Geometry check sheet. Reference: the model listing, model coordinates, mm. Face numbers are marked on the shaded views. A direction names the side the tool comes from. Round coordinates to 2 decimals unless told otherwise and drop trailing zeros. Order: outer loops, then holes, each group sorted by start corner. A loop starts at its lowest first (then second) coordinate and runs counter-clockwise, first axis right, second up. Notation, with made-up numbers: M 21.5,42.5 L 49.5,42.5 A15 ccw 49.5,52.5 Z; hole C 11.5,-26 d1. An arc over 180 degrees is marked long. Return JSON: item names as keys, results as strings. Group by question number.
```python
from build123d import *

# Parameters (mm, degrees)
SKETCH1_W               = 41.91
SKETCH1_H               = 82.55
BOSS_EXTRUDE1_DEPTH     = 58.674
SKETCH2_R               = 20.32
BOSS_EXTRUDE2_DEPTH     = 76.2
SKETCH3_R               = 18.415
BOSS_EXTRUDE3_DEPTH     = 101.6
SKETCH4_R               = 9.9949
BOSS_EXTRUDE4_DEPTH     = 19.05
CUT_EXTRUDE1_DEPTH      = 19.05
CUT_EXTRUDE1_DEPTH_BACK = 19.05
SKETCH6_R               = 3.175
SKETCH7_W               = 18
SKETCH7_H               = 18
BOSS_EXTRUDE5_DEPTH     = 20
CUT_EXTRUDE2_DEPTH      = 20
CUT_EXTRUDE2_DEPTH_BACK = 20
SKETCH8_R               = 3.175


with BuildPart() as part:
    # Sketch1 → Boss-Extrude1 (new body)
    with BuildSketch(Plane.XY):
        with Locations((0, 41.275)):
            Rectangle(SKETCH1_W, SKETCH1_H)
    extrude(amount=BOSS_EXTRUDE1_DEPTH)

    # Sketch2 → Boss-Extrude2 (add)
    with BuildSketch(Plane.XY.offset(58.674)):
        with Locations(Location((0, 62.23, 0), (0, 0, 90))):
            Circle(SKETCH2_R)
    extrude(amount=BOSS_EXTRUDE2_DEPTH)

    # Sketch3 → Boss-Extrude3 (add)
    with BuildSketch(Plane.XY.offset(58.674)):
        with Locations(Location((0, 19.05, 0), (0, 0, 180))):
            Circle(SKETCH3_R)
    extrude(amount=BOSS_EXTRUDE3_DEPTH)

    # Sketch4 → Boss-Extrude4 (add)
    with BuildSketch(Plane.XY.offset(160.274)):
        with Locations(Location((0, 22.225, 0), (0, 0, 180))):
            Circle(SKETCH4_R)
    extrude(amount=BOSS_EXTRUDE4_DEPTH)

    # Sketch6 → Cut-Extrude1 (cut, two sides: drawn at the far end of the back side and taken through both)
    with BuildSketch(Plane(origin=(0, 0, 0), x_dir=(0, 0, -1), z_dir=(1, 0, 0)).offset(-CUT_EXTRUDE1_DEPTH_BACK)):
        with Locations(Location((-170.324, 22.225, 0), (0, 0, 180))):
            Circle(SKETCH6_R)
    extrude(amount=CUT_EXTRUDE1_DEPTH + CUT_EXTRUDE1_DEPTH_BACK, mode=Mode.SUBTRACT)

    # Sketch7 → Boss-Extrude5 (add)
    with BuildSketch(Plane(origin=(0, 0, 0), x_dir=(-1, 0, 0), z_dir=(0, 0, -1))):
        with Locations((0, 24)):
            Rectangle(SKETCH7_W, SKETCH7_H)
    extrude(amount=BOSS_EXTRUDE5_DEPTH)

    # Sketch8 → Cut-Extrude2 (cut, two sides: drawn at the far end of the back side and taken through both)
    with BuildSketch(Plane.ZY.offset(9).offset(-CUT_EXTRUDE2_DEPTH_BACK)):
        with Locations(Location((-12, 24, 0), (0, 0, 180))):
            Circle(SKETCH8_R)
    extrude(amount=CUT_EXTRUDE2_DEPTH + CUT_EXTRUDE2_DEPTH_BACK, mode=Mode.SUBTRACT)


solid = part.part
```
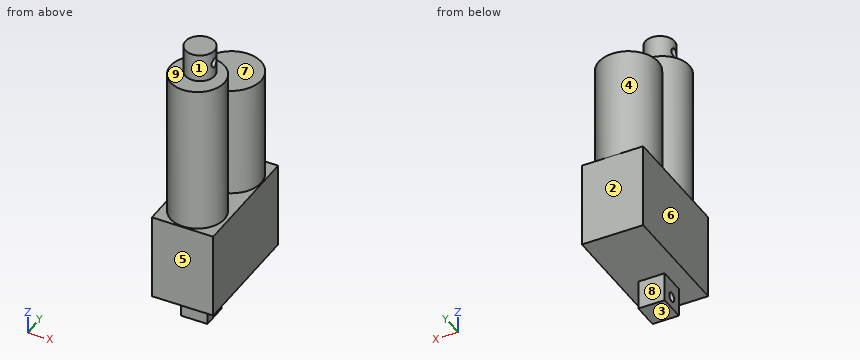
Q1. Section check A-A on z = -12. Record the cut outline in (x, y) (3 decimals), plus the area to 3 significant figures.
Q2. Section check C-C on y = 62.23. Record the cut outline in (x, z) (3 decimals), plus the area to 3 significant figures.
Q3. Depth check by flat-ended pin: pin 1 Ø5.5 at (y, z) = (22.5, -6) entering from +X; pin 2 Ø5 at (y, z) = (43, 91.5) entering from +X; pin 3 Ø2 at (x, y) = (12.5, 68.5) entering from +Z. Enter the tip coordinate at first touch or a pass-through.
Q4. Section check D-D on y = 45. Record the cut outline in (x, z) (3 decimals), plus the area to 3 significant figures.
Q5. Release check for a two-part mould opening along Y. For the marked faces 1, 2, 3 and 4 record: +Y half, -Y half, draft (parallel to the pull), parting line (faces both ways), or undercut.
Q6. Section check B-B on x = 2.5. Record the cut outline in (y, z) (3 decimals), plus the area to 3 significant figures.
Q7. Material ranges on line 1 along X through (y, z) = (62.5, 106); line 2 along Z through (x, y) = (8.5, 52.5); line 3 along Y through (x, z) = (0, -12) (3 decimals), recorded low to high.
Q8. Set-up check for the marked faces 5, 6, 7, 8 and 9: record each of +Z, -Z, +X, -X, +Y, -Y from which the full face is reachable in a straight line by a thin tool's end or side.
Geometry check:
{
 "1": {"outline": "M -9,15 L 9,15 L 9,20.825 L -9,20.825 Z; M -9,27.175 L 9,27.175 L 9,33 L -9,33 Z", "area": "210 mm^2"},
 "2": {"outline": "M -20.955,0 L 20.955,0 L 20.955,58.674 L 20.32,58.674 L 20.32,134.874 L -20.32,134.874 L -20.32,58.674 L -20.955,58.674 Z", "area": "5,560 mm^2"},
 "3": {"pin 1": "stops at x = 9", "pin 2": "stops at x = 11.53", "pin 3": "stops at z = 134.87"},
 "4": {"outline": "M -20.955,0 L 20.955,0 L 20.955,58.674 L 10.772,58.674 L 10.772,134.874 L -10.772,134.874 L -10.772,58.674 L -20.955,58.674 Z", "area": "4,100 mm^2"},
 "5": {"face 1": "parting line", "face 2": "+Y half", "face 3": "draft", "face 4": "undercut"},
 "6": {"outline": "M 0,0 L 15,0 L 15,-20 L 33,-20 L 33,0 L 82.55,0 L 82.55,58.674 L 82.396,58.674 L 82.396,134.874 L 42.064,134.874 L 42.064,58.674 L 37.295,58.674 L 37.295,160.274 L 31.902,160.274 L 31.902,179.324 L 12.548,179.324 L 12.548,160.274 L 0.805,160.274 L 0.805,58.674 L 0,58.674 Z; hole C 22.225,170.324 d6.35; hole C 24,-12 d6.35", "area": "12,300 mm^2"},
 "7": {"line 1": "x = -20.32 to 20.32", "line 2": "z = 0 to 134.87", "line 3": "y = 15 to 20.825, 27.175 to 33"},
 "8": {"face 5": "+Z, -Z, +X, -X, -Y", "face 6": "+Z, -Z, -X, +Y, -Y", "face 7": "+Z, +X, -X, +Y", "face 8": "-Z, +X, -X, +Y", "face 9": "+Z"}
}
